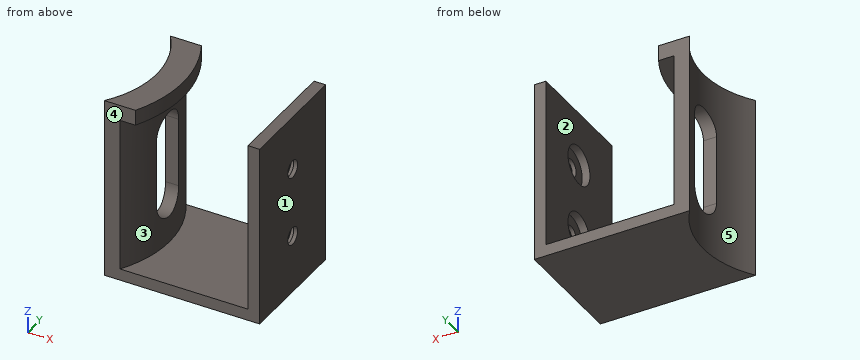
Autodesk Inventor part; units mm, degrees
ref_plane "YZ Plane" through (0, 0, 0) normal (1, 0, 0) x (0, 1, 0)
ref_plane "XZ Plane" through (0, 0, 0) normal (0, 1, 0) x (-1, 0, 0)
ref_plane "XY Plane" through (0, 0, 0) normal (0, 0, 1) x (1, 0, 0)
sketch "Sketch1" plane through (0, 0, 0) normal (1, 0, 0) x (0, 1, 0)
  line L0 (-15, -15) -> (15, -15)
  line L1 (15, -15) -> (15, 15)
  line L2 (15, 15) -> (-15, 15)
  line L3 (-15, 15) -> (-15, -15)
  line L4 (-15, -15) -> (15, 15) construction
  line L5 (15, -15) -> (-15, 15) construction
  point P0 (0, 0)
  dimension "d0" = 30
  dimension "d1" = 30
extrude "Extrusion1" add sketch "Sketch1" along normal blind 3
sketch "Sketch2" plane through (0, -15, -15) normal (0, 0, -1) x (-1, 0, 0)
  line L0 (0, 30) -> (-3, 30)
  line L1 (-3, 30) -> (37, 30)
  line L2 (37, 30) -> (37, 0)
  line L3 (37, 0) -> (-3, 0)
  line L4 (-3, 0) -> (-3, 30)
  point P0 (0, 15)
  dimension "d4" = 40
  dimension "d5" = 30
extrude "Extrusion2" add sketch "Sketch2" along normal blind 3
sketch "Sketch3" plane through (0, -15, -15) normal (0, 0, 1) x (1, 0, 0)
  line L0 (0, 0) -> (-37, 0)
  line L1 (-37, 0) -> (-37, 30)
  arc A0 (-37, 0) -> (-37, 30) centre (-57.325, 15) ccw
  point P0 (0, 15)
extrude "Extrusion3" cut sketch "Sketch3" against normal blind 3
sketch "Sketch4" plane through (0, -15, -15) normal (0, 0, 1) x (1, 0, 0)
  line L0 (-37, 30) -> (0, 30)
  arc A0 (-37, 0) -> (-37, 30) centre (-57.325, 15) ccw
  line L1 (-33.6755, 30) -> (-37, 30)
  point P0 (0, 15)
sketch "Sketch5" plane through (0, -15, -15) normal (0, 0, 1) x (1, 0, 0)
  arc A0 (-37, 0) -> (-37, 30) centre (-57.325, 15) ccw
  line L0 (-37, 30) -> (-33, 30)
  line L1 (-37, 30) -> (0, 30)
  line L2 (0, 0) -> (-37, 0)
  arc A1 (-33, 0) -> (-33, 30) centre (-57.325, 15) ccw
  line L3 (-33, 0) -> (-37, 0)
  arc A2 (-37, 0) -> (-37, 30) centre (-57.325, 15) ccw
  point P0 (0, 15)
  dimension "d10" = 4
extrude "Extrusion4" add sketch "Sketch5" along normal blind 40
sketch "Sketch6" plane through (0, -15, 25) normal (0, 0, 1) x (1, 0, 0)
  line L0 (-33, 30) -> (-37, 30)
  line L1 (-37, 30) -> (-29, 30)
  arc A0 (-37, 0) -> (-37, 30) centre (-57.325, 15) ccw
  line L2 (-37, 0) -> (-29, 0)
  arc A1 (-29, 0) -> (-29, 30) centre (-57.325, 15) ccw
  arc A2 (-37, 0) -> (-37, 30) centre (-57.325, 15) ccw
  point P0 (0, 15)
  dimension "d13" = 8
extrude "Extrusion5" add sketch "Sketch6" along normal blind 4
sketch "Sketch7" plane through (0, -15, 15) normal (0, -1, 0) x (1, 0, 0)
  point P0 (0, -15)
sketch "Sketch8" plane through (0, -15, 15) normal (0, 0, 1) x (1, 0, 0)
  point P0 (0, 15)
sketch "Sketch9" plane through (0, -15, 15) normal (0, -1, 0) x (1, 0, 0)
  line L0 (3, 0) -> (3, -33)
  line L1 (3, 0) -> (3, 14)
  line L2 (3, 14) -> (0, 14)
  line L3 (0, 0) -> (3, 0)
  line L4 (0, 14) -> (0, 0)
  line L5 (0, 0) -> (3, 0)
  point P0 (0, -15)
  dimension "d16" = 14
extrude "Extrusion6" add sketch "Sketch9" against normal blind 30
sketch "Sketch10" plane through (0, 0, 0) normal (-1, 0, 0) x (0, 0, 1)
  point P0 (0, 0)
sketch "Sketch11" plane through (0, 0, 0) normal (-1, 0, 0) x (0, 0, 1)
  arc A0 (14.9299, -5.0174) -> (14.976, 4.9821) centre (15, -0.0179) ccw
  arc A1 (-2.9259, 4.9821) -> (-3, -5.0174) centre (-3, -0.0174) ccw
  line L0 (-15, -15) -> (-15, 15)
  line L1 (29, -15) -> (29, 15)
  line L2 (14.9299, -5.0174) -> (-3, -5.0174)
  line L3 (15.024, 4.9821) -> (-3.0741, 4.9821)
  line L4 (29, -15) -> (-15, -15)
  line L5 (-15, 15) -> (29, 15)
  point P0 (0, 0)
  point P1 (-15, 0)
  point P2 (29, 0)
  dimension "d19" = 10
  dimension "d20" = 10
  dimension "d21" = 12
  dimension "d22" = 14
extrude "Extrusion7" cut sketch "Sketch11" along normal blind 50 contours L2 A1 L3 A0
sketch "Sketch12" plane through (0, 0, 0) normal (-1, 0, 0) x (0, 0, 1)
  circle A0 centre (-3, 0) radius 5
  circle A1 centre (15, 0) radius 5
  line L0 (29, -15) -> (29, 15)
  line L1 (-15, -15) -> (-15, 15)
  point P0 (0, 0)
  point P1 (29, 0)
  point P2 (-15, 0)
  dimension "d25" = 10
  dimension "d26" = 10
  dimension "d27" = 14
  dimension "d28" = 12
extrude "Extrusion8" cut sketch "Sketch12" against normal blind 2
sketch "Sketch13" plane through (2, 0, 15) normal (-1, 0, 0) x (0, 0, 1)
  circle A0 centre (0, 0) radius 2.25
  circle A1 centre (-18, 0) radius 2.25
  circle A2 centre (-18, 0) radius 5
  point P0 (-15, 0)
  dimension "d31" = 4.5
  dimension "d32" = 4.5
  dimension "d33" = 2.75
extrude "Extrusion9" cut sketch "Sketch13" against normal blind 3 contours A0 | A1
sketch "Sketch14" plane through (3, 0, 0) normal (1, 0, 0) x (0, 0, -1)
  line L0 (-29, 15) -> (18, 15)
  line L1 (-29, -15) -> (18, -15)
  line L2 (-29, 15) -> (18, 15)
  line L3 (18, 15) -> (18, -15)
  line L4 (18, -15) -> (-29, -15)
  line L5 (-29, -15) -> (-29, 15)
  circle A0 centre (3, 0) radius 2.25
  circle A1 centre (3, 0) radius 5
  circle A2 centre (-15, 0) radius 5
  circle A3 centre (-15, 0) radius 5
  point P0 (0, 0)
properties part number "headphones_hook1.1"
Read the model definition and answer for the solid it produces. Units are mm, in the model's axes. Face numbers are marked on the shaded views. A direction names the side the tool comes from. Give positions to 0.01 mm unless a question says otherwise; leave off trailing zeros. Loops run counter-clockwise (first coordinate to the right, second up) from the corner with the lowest first, then second, coordinate; pieces in that order, holes last.
Item 1: Find the intervals of material crossed by line 1 along Y through (x, z) = (2.4, -3); line 2 along Z through (x, y) = (-14.5, 0.5); line 3 along Y through (x, z) = (1.5, 15), in increasing order.
Item 2: The mould has two halves that part along X. Classify the marked faces 3, 4 and 5: released by +X, released by -X, zero draft, split by the parting line, or undercut.
Item 3: For the marked faces 1 and 2, determine the directions among +Z, -Z, +X, -X, +Y, -Y from which every point of the face is accessible in a straight line to the end or side of a thin tool.
Item 4: The part is cut by section B-B (y = -4). Write down the section's boundary in (x, z).
Item 5: Each of these flat-tipped pins is pushed along its axis until it touches: pin 1 Ø11 at (y, z) = (-2, -3.5) entering from -X; pin 2 Ø5 at (y, z) = (2, 14) entering from -X; pin 3 Ø3.5 at (x, z) = (-30.5, 8.5) entering from -Y. Where does it stop, or does it pass through?
Item 6: The part is cut by section A-A (z = 23.5). Write down the section's boundary in (x, y) (1 decimal), and give its area (3 significant figures).
Item 7: The part is cut by section D-D (y = 12). Write down the section's boundary in (x, z).
Item 8: The part is cut by section C-C (y = 0). Give the number of separate pieces and of enclosed holes in the cut face, and give its area (3 significant figures).
Taken from the geometry:
1. line 1: y = -15 to -2.25, 2.25 to 15
1. line 2: z = -18 to -15
1. line 3: y = -15 to -5, 5 to 15
2. face 3: undercut
2. face 4: zero draft
2. face 5: released by -X
3. face 1: +Z, -Z, +X, +Y, -Y
3. face 2: +Z, +Y, -Y
4. outline: (-32.38, -18) - (3, -18) - (3, 29) - (0, 29) - (0, 18) - (2, 18) - (2, 12) - (0, 12) - (0, 0) - (2, 0) - (2, -6) - (0, -6) - (0, -15) - (-29.03, -15) - (-29.03, -6.02) - (-32.38, -6.02) - close; (-32.38, 18.02) - (-29.03, 18.02) - (-29.03, 25) - (-25.52, 25) - (-25.52, 29) - (-32.38, 29) - close
5. pin 1: stops at x = -33.2
5. pin 2: stops at x = 2
5. pin 3: stops at y = -13.71
6. outline: (-37, -15) - (-33, -15) arc R28.6 ccw to (-33, 15) - (-37, 15) arc R25.3 cw to start; (0, -15) - (3, -15) - (3, 15) - (0, 15) - close
6. area: 196 mm2
7. outline: (-35.1, -18) - (3, -18) - (3, 29) - (0, 29) - (0, -15) - (-31.39, -15) - (-31.39, 25) - (-27.6, 25) - (-27.6, 29) - (-35.1, 29) - close
8. separate pieces: 4
8. enclosed holes: 0
8. area: 255 mm2
